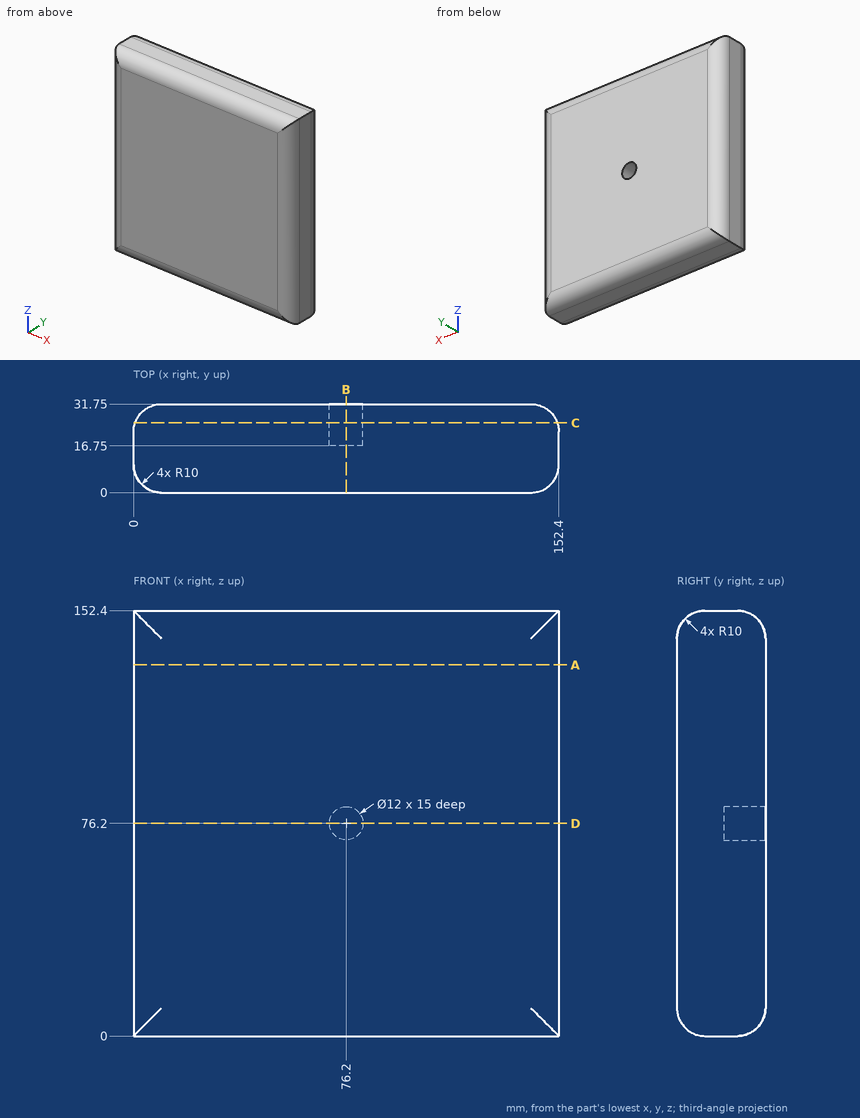
Can you work these out from the drawing? Everything is in mm from the part's minimum corner. Give positions to 0.01 mm unless a question says otherwise; leave off trailing zeros. Order: outer loops, then holes, each group sorted by start corner. A loop starts at its lowest first (then second) coordinate and runs counter-clockwise, first axis right, second up. Notation, with made-up numbers: M 81.5,-2.75 L 136.5,-2.75 A35 ccw 136.5,34.25 Z; hole C -8.75,35 d1. An arc over 180 degrees is marked long. Use a Markdown table: item, result. Add a question column.
Item 1: Will these pins go through, and if not, where does the flat tip stop? pin 1 (8 mm diameter, centred on x = 77.5, y = 25, fed in from -Z); pin 2 (6 mm diameter, centred on x = 78, z = 74, fed in from +Y); pin 3 (1 mm diameter, centred on x = 67.5, y = 23.5, fed in from +Z).
Item 2: Suppose I cut it at B-B (x = 76.2). List the corners of the cut face in (y, z) for me, then the cut area to 3 significant figures.
Item 3: If I drill on L1, parallel to X at y = 22.25, z = 76.2; L2, parallel to X at y = 27.75, z = 76.2; L3, parallel to Z at x = 29.5, y = 22.5, over which ranges is the centre line in solid material (lowest first)? Write a range as [from, to].
Item 4: Suppose I cut it at A-A (z = 133). List the corners of the cut face in (x, y) for me.
Item 5: Suppose I cut it at D-D (z = 76.2). List the corners of the cut face in (x, y) for me, then the cut area to 3 significant figures.
Item 6: Suppose I cut it at C-C (y = 25). List the corners of the cut face in (x, z) for me, then the cut area to 3 significant figures.
Answer sheet:
| question | item | result |
|---|---|---|
| 1 | pin 1 | stops at z = 0 |
| 1 | pin 2 | stops at y = 16.75 |
| 1 | pin 3 | stops at z = 152.32 |
| 2 | outline | M 0,10 A10 ccw 10,0 L 21.75,0 A10 ccw 31.75,10 L 31.75,70.2 L 16.75,70.2 L 16.75,82.2 L 31.75,82.2 L 31.75,142.4 A10 ccw 21.75,152.4 L 10,152.4 A10 ccw 0,142.4 Z |
| 2 | area | 4,570 mm² |
| 3 | L1 | x = [0.01, 70.2], [82.2, 152.39] |
| 3 | L2 | x = [2, 70.2], [82.2, 150.4] |
| 3 | L3 | z = [0.03, 152.37] |
| 4 | outline | M 0,10 A10 ccw 10,0 L 142.4,0 A10 ccw 152.4,10 L 152.4,21.75 A10 ccw 142.4,31.75 L 10,31.75 A10 ccw 0,21.75 Z |
| 5 | outline | M 0,10 A10 ccw 10,0 L 142.4,0 A10 ccw 152.4,10 L 152.4,21.75 A10 ccw 142.4,31.75 L 82.2,31.75 L 82.2,16.75 L 70.2,16.75 L 70.2,31.75 L 10,31.75 A10 ccw 0,21.75 Z |
| 5 | area | 4,570 mm² |
| 6 | outline | M 0.54,0.54 L 151.86,0.54 L 151.86,151.86 L 0.54,151.86 Z; hole C 76.2,76.2 d12 |
| 6 | area | 22,800 mm² |
